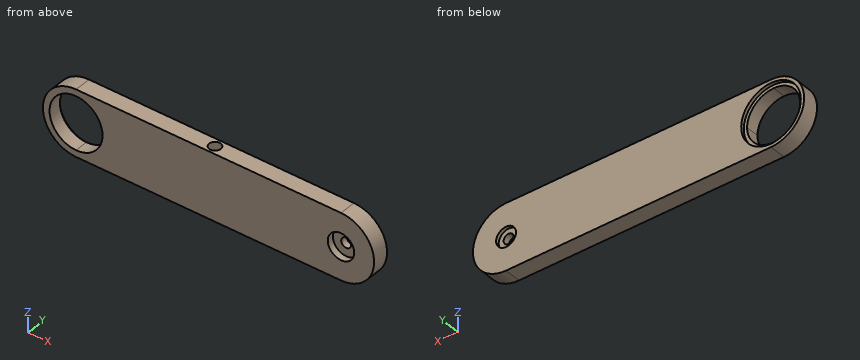
```python
from build123d import *

# Parameters (mm, degrees)
BOSS_EXTRUDE1_DEPTH = 5
CUT_EXTRUDE1_DEPTH  = 52.23475383
SKETCH3_R           = 9
CUT_EXTRUDE2_DEPTH  = 1
SKETCH4_R           = 3
CUT_EXTRUDE3_DEPTH  = 1
SKETCH5_R           = 1.5
CUT_EXTRUDE4_DEPTH  = 52.14684741
SKETCH6_R           = 4
CUT_EXTRUDE5_DEPTH  = 2
SKETCH8_R           = 1.75
CUT_EXTRUDE7_DEPTH  = 10


with BuildPart() as part:
    # Sketch1 → Boss-Extrude1 (new body)
    with BuildSketch(Plane(origin=(0, 0, 0), x_dir=(1, 0, 0), z_dir=(0, 1, 0))):
        with BuildLine():
            Line((-40, 10), (40, 10))
            ThreePointArc((40, 10), (50, 0), (40, -10))
            Line((40, -10), (-40, -10))
            ThreePointArc((-40, -10), (-50, 0), (-40, 10))
        make_face()
    extrude(amount=BOSS_EXTRUDE1_DEPTH)

    # Sketch2 → Cut-Extrude1 (cut, through all)
    with BuildSketch(Plane(origin=(0, 5, 0), x_dir=(1, 0, 0), z_dir=(0, 1, 0))):
        with BuildLine():
            ThreePointArc((-32, 0), (-34.343145751, 5.656854249), (-40, 8))
            Line((-40, 8), (-40, -8))
            ThreePointArc((-40, -8), (-34.343145751, -5.656854249), (-32, 0))
        make_face()
        with BuildLine():
            Line((-40, -8), (-40, 8))
            ThreePointArc((-40, 8), (-48, 0), (-40, -8))
        make_face()
    extrude(amount=-CUT_EXTRUDE1_DEPTH, mode=Mode.SUBTRACT)

    # Sketch3 → Cut-Extrude2 (cut)
    with BuildSketch(Plane(origin=(0, 5, 0), x_dir=(1, 0, 0), z_dir=(0, 1, 0))):
        with Locations(Location((-40, 0, 0), (0, 0, 270))):
            Circle(SKETCH3_R)
    extrude(amount=-CUT_EXTRUDE2_DEPTH, mode=Mode.SUBTRACT)

    # Sketch4 → Cut-Extrude3 (cut)
    with BuildSketch(Plane(origin=(0, 5, 0), x_dir=(1, 0, 0), z_dir=(0, 1, 0))):
        with Locations(Location((40, 0, 0), (0, 0, 270))):
            Circle(SKETCH4_R)
    extrude(amount=-CUT_EXTRUDE3_DEPTH, mode=Mode.SUBTRACT)

    # Sketch5 → Cut-Extrude4 (cut, through all)
    with BuildSketch(Plane(origin=(0, 4, 0), x_dir=(1, 0, 0), z_dir=(0, 1, 0))):
        with Locations(Location((40, 0, 0), (0, 0, 270))):
            Circle(SKETCH5_R)
    extrude(amount=-CUT_EXTRUDE4_DEPTH, mode=Mode.SUBTRACT)

    # Sketch6 → Cut-Extrude5 (cut)
    with BuildSketch(Plane.XZ):
        with Locations(Location((40, 0, 0), (0, 0, 270))):
            Circle(SKETCH6_R)
    extrude(amount=-CUT_EXTRUDE5_DEPTH, mode=Mode.SUBTRACT)

    # Sketch8 → Cut-Extrude7 (cut)
    with BuildSketch(Plane.XY.offset(10)):
        with Locations((0, 2.5)):
            Circle(SKETCH8_R)
    extrude(amount=-CUT_EXTRUDE7_DEPTH, mode=Mode.SUBTRACT)


solid = part.part
```
Check sheet for the modelled part. Datum: model origin and axes. Units: mm. Coordinates: 2 decimals unless noted, no trailing zeros. Write each loop counter-clockwise with the first axis right and the second up, starting at its lowest first coordinate (ties: lowest second). Pieces come first, ordered by that corner, then holes. Notation, with made-up numbers: M 87,4.25 L 98,4.25 A24 cw 98,32.25 Z; hole C 49,12 d8. An arc over 180 degrees is marked long. Write item = value, one per line. Start each with the question number.
1. Go/stop test with flat-tipped pins: pin 1 (5 mm diameter, centred on x = -27, z = 5.5, fed in from -Y); pin 2 (2.5 mm diameter, centred on x = 38, z = -1, fed in from -Y); pin 3 (4 mm diameter, centred on x = 40, z = 0, fed in from +Y). Record where each tip stops, or that it passes through.
2. Sectioned sample at C-C (x = 0). Record the cut outline in (y, z), then the cut area to 3 significant figures.
3. Sectioned sample at A-A (z = 6). Record the cut outline in (x, y).
4. Sectioned sample at D-D (z = -5.25). Record the cut outline in (x, y), then the cut area to 3 significant figures.
5. Thickness scan on probe 1 along X at (y, z) = (4.7, 0); probe 2 along X at (y, z) = (1.55, -3.5); probe 3 along Y at (x, z) = (42, -0.5). Record the ranges inside material, lowest first.
6. Sectioned sample at B-B (x = -43.5). Record the cut outline in (y, z), then the cut area to 3 significant figures.
The answers:
q1.pin_1 = 0
q1.pin_2 = 2
q1.pin_3 = 4
q2.outline = M 0,-10 L 5,-10 L 5,10 L 4.25,10 L 4.25,0 L 0.75,0 L 0.75,10 L 0,10 Z
q2.area = 65.0 mm²
q3.outline = M -48,0 L -45.29,0 L -45.29,4 L -46.71,4 L -46.71,5 L -48,5 Z; M -34.71,0 L 48,0 L 48,5 L -33.29,5 L -33.29,4 L -34.71,4 Z; hole C 0,2.5 d3.5
q4.outline = M -48.51,0 L -46.04,0 L -46.04,4 L -47.31,4 L -47.31,5 L -48.51,5 Z; M -33.96,0 L 48.51,0 L 48.51,5 L -32.69,5 L -32.69,4 L -33.96,4 Z
q4.area = 422 mm²
q5.probe_1 = -50 to -49, -31 to 37, 43 to 50
q5.probe_2 = -49.37 to -47.19, -32.81 to 38.06, 41.94 to 49.37
q5.probe_3 = 2 to 4
q6.outline = M 0,-9.37 L 5,-9.37 L 5,-8.29 L 4,-8.29 L 4,-7.19 L 0,-7.19 Z; M 0,7.19 L 4,7.19 L 4,8.29 L 5,8.29 L 5,9.37 L 0,9.37 Z
q6.area = 19.5 mm²
